Geometry: final body of the model. Coordinates: model frame, mm. Give positions to 0.01 mm unless a question says otherwise; leave off trailing zeros. Order: outer loops, then holes, each group sorted by start corner. A loop starts at its lowest first (then second) coordinate and runs counter-clockwise, first axis right, second up. Notation, with made-up numbers: (-12, 8.25) -> (13, 8.25) arc R25 cw to (13, 24.25) -> close; hole circle Ø6 at (32.5, 9.25). An arc over 180 degrees is marked (long way). Write item = value, one per line.
```python
from build123d import *

# Parameters (mm, degrees)
F0_R     = 127
F0_R_2   = 37.1475
F1_DEPTH = 19.05
F3_DEPTH = 25.4


with BuildPart() as f1:
    # F0 (on Front) → F1 (new body)
    with BuildSketch(Plane.XZ):
        Circle(F0_R)
        Circle(F0_R_2, mode=Mode.SUBTRACT)
    extrude(amount=F1_DEPTH)

    # F2 (on face) → F3 (cut)
    with BuildSketch(Plane(origin=(0, 0, 0), x_dir=(-1, 0, 0), z_dir=(0, 1, 0))):
        with BuildLine():
            ThreePointArc((-17.584615, 74.143249), (-14.06865, 76.38375), (-12.7, 80.321853))
            Line((-12.7, 80.321853), (-12.7, 93.325559))
            ThreePointArc((-12.7, 93.325559), (-15.033907, 98.244248), (-20.32, 99.547263))
            ThreePointArc((-20.32, 99.547263), (-71.842049, 71.842049), (-99.547263, 20.32))
            ThreePointArc((-99.547263, 20.32), (-98.244248, 15.033907), (-93.325559, 12.7))
            Line((-93.325559, 12.7), (-80.321853, 12.7))
            ThreePointArc((-80.321853, 12.7), (-76.38375, 14.06865), (-74.143249, 17.584615))
            ThreePointArc((-74.143249, 17.584615), (-53.881537, 53.881537), (-17.584615, 74.143249))
        make_face()
        with BuildLine():
            ThreePointArc((17.584615, 74.143249), (53.881537, 53.881537), (74.143249, 17.584615))
            ThreePointArc((74.143249, 17.584615), (76.38375, 14.06865), (80.321853, 12.7))
            Line((80.321853, 12.7), (93.325559, 12.7))
            ThreePointArc((93.325559, 12.7), (98.244248, 15.033907), (99.547263, 20.32))
            ThreePointArc((99.547263, 20.32), (71.842049, 71.842049), (20.32, 99.547263))
            ThreePointArc((20.32, 99.547263), (15.033907, 98.244248), (12.7, 93.325559))
            Line((12.7, 93.325559), (12.7, 80.321853))
            ThreePointArc((12.7, 80.321853), (14.06865, 76.38375), (17.584615, 74.143249))
        make_face()
        with BuildLine():
            Line((93.325559, -12.7), (80.321853, -12.7))
            ThreePointArc((80.321853, -12.7), (76.38375, -14.06865), (74.143249, -17.584615))
            ThreePointArc((74.143249, -17.584615), (53.881537, -53.881537), (17.584615, -74.143249))
            ThreePointArc((17.584615, -74.143249), (14.06865, -76.38375), (12.7, -80.321853))
            Line((12.7, -80.321853), (12.7, -93.325559))
            ThreePointArc((12.7, -93.325559), (15.033907, -98.244248), (20.32, -99.547263))
            ThreePointArc((20.32, -99.547263), (71.842049, -71.842049), (99.547263, -20.32))
            ThreePointArc((99.547263, -20.32), (98.244248, -15.033907), (93.325559, -12.7))
        make_face()
        with BuildLine():
            ThreePointArc((-74.143249, -17.584615), (-76.38375, -14.06865), (-80.321853, -12.7))
            Line((-80.321853, -12.7), (-93.325559, -12.7))
            ThreePointArc((-93.325559, -12.7), (-98.244248, -15.033907), (-99.547263, -20.32))
            ThreePointArc((-99.547263, -20.32), (-71.842049, -71.842049), (-20.32, -99.547263))
            ThreePointArc((-20.32, -99.547263), (-15.033907, -98.244248), (-12.7, -93.325559))
            Line((-12.7, -93.325559), (-12.7, -80.321853))
            ThreePointArc((-12.7, -80.321853), (-14.06865, -76.38375), (-17.584615, -74.143249))
            ThreePointArc((-17.584615, -74.143249), (-53.881537, -53.881537), (-74.143249, -17.584615))
        make_face()
    extrude(amount=-F3_DEPTH, mode=Mode.SUBTRACT)


solid = f1.part
```
1) Section query B-B (z = 0). Output: boundary loops of the cut face in (x, y).
Check sheet entries:
outline = (-127, -19.05) -> (-37.15, -19.05) -> (-37.15, 0) -> (-127, 0) -> close; (37.15, -19.05) -> (127, -19.05) -> (127, 0) -> (37.15, 0) -> close
2) Line query: line 1 (Z direction, x = 0, y = -5); line 2 (X direction, y = -16.25, z = 81); line 3 (X direction, y = -10, z = -93). Output: solid intervals per line, ascending. Write a range as from..to.
Check sheet entries:
line_1 = -127..-37.15, 37.15..127
line_2 = -97.82..-61.33, -12.7..12.7, 61.33..97.82
line_3 = -86.49..-40.91, -12.7..12.7, 40.91..86.49
3) Mould query, pull axis X, two halves, no side actions, for faces 1 (the face through (-27.53, -9.39, -123.98)), 2 (the face through (-71.25, -9.39, -72.43)). Classes: +X half, -X half, draft (parallel to the pull), parting line (faces both ways), or undercut.
Check sheet entries:
face_1 = parting line
face_2 = undercut
4) Section query C-C (y = -9). Count the separate pieces of the cut face and the enclosed holes in it, plus the area to 3 significant figures.
Check sheet entries:
separate_pieces = 1
enclosed_holes = 5
area = 34,900 mm²
5) Section query D-D (z = 69). Output: boundary loops of the cut face in (x, y), plus the area to 3 significant figures.
Check sheet entries:
outline = (-106.62, -19.05) -> (-74.58, -19.05) -> (-74.58, 0) -> (-106.62, 0) -> close; (-32.33, -19.05) -> (32.33, -19.05) -> (32.33, 0) -> (-32.33, 0) -> close; (74.58, -19.05) -> (106.62, -19.05) -> (106.62, 0) -> (74.58, 0) -> close
area = 2,450 mm²
6) First-contact query: P1, Ø4, axis at y = -9.5, z = -86.5, coming from the +X side; P2, Ø10.5, axis at y = -5.5, z = -87.5, coming from the -X side; P3, Ø6, axis at x = -31, y = -4.5, coming from the -Z side. Flat tips, straight axial feed; report the tip coordinate or a pass-through.
Check sheet entries:
P1 = 94.81
P2 = -96.77
P3 = -123.87
7) Section query A-A (x = 0). Output: boundary loops of the cut face in (y, z).
Check sheet entries:
outline = (-19.05, -127) -> (0, -127) -> (0, -37.15) -> (-19.05, -37.15) -> close; (-19.05, 37.15) -> (0, 37.15) -> (0, 127) -> (-19.05, 127) -> close
